Check sheet for the drawn part. Datum: minimum x, y, z corner. Units: mm. A direction names the side the tool comes from. Coordinates: 2 decimals unless noted, no trailing zeros. Write each loop counter-clockwise with the first axis right and the second up, starting at its lowest first coordinate (ties: lowest second). Pieces come first, ordered by that corner, then holes. Notation, with made-up numbers: (67.25, 63.5) - (96.25, 63.5) arc R17 ccw to (96.25, 84.5) - close; hole circle Ø6 at (63.25, 17.5). An arc over 180 degrees is marked (long way). Use CSV: the item, a comma, the result in double quotes. Start each with the question number.
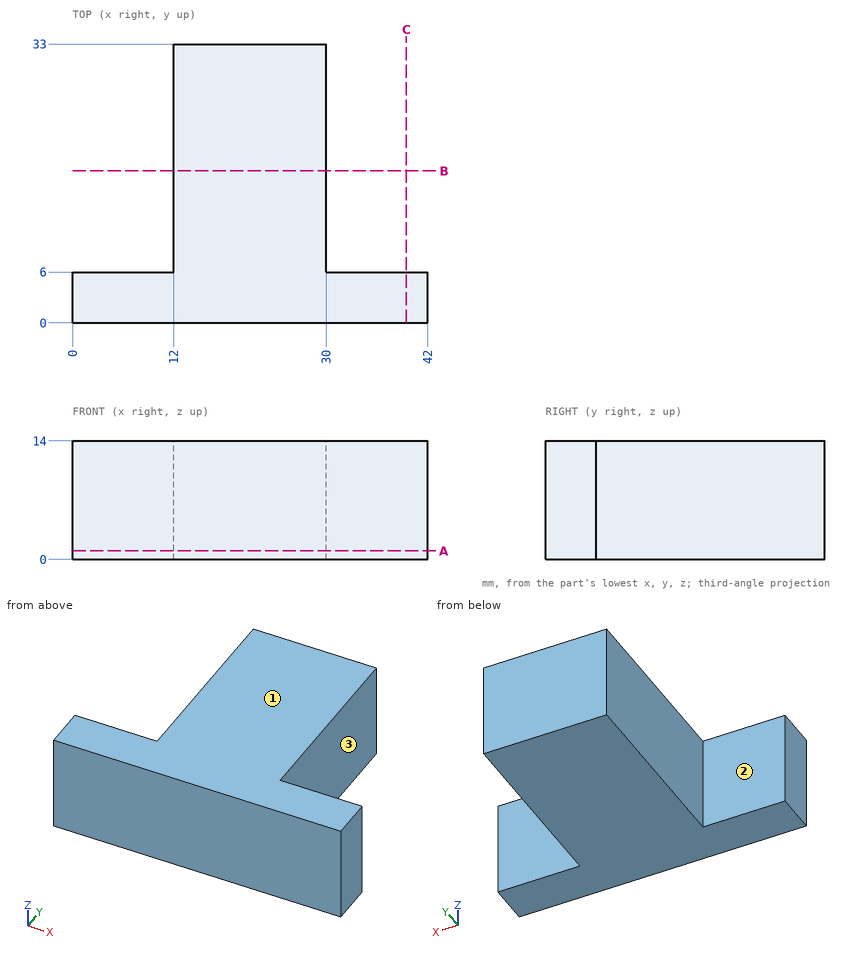
Q1. Scan lines: line 1 along Y through (x, z) = (3, 7); line 2 along X through (y, z) = (10.5, 3). Record each from-to range of solid material in increasing order. Write a range as from..to.
Q2. Gauge pin test, flat ends, axial feed: pin 1 (5 mm diameter, centred on x = 9, y = 24, fed in from +Z); pin 2 (2 mm diameter, centred on y = 19, z = 9, fed in from +X); pin 3 (3.5 mm diameter, centred on x = 9, z = 6.5, fed in from +Y). Record the tip position at first contact, or that the pin passes through.
Q3. Cross-section at C-C (x = 39.5). Record the cut outline in (y, z).
Q4. Tool access check on the marked faces 1, 2 and 3. Record the directions out of +Z, -Z, +X, -X, +Y, -Y that give a thin tool (end or side, any length) a straight path to the whole face; none if there is none.
Q5. Cross-section at B-B (y = 18). Record the cut outline in (x, z).
Q6. Cross-section at A-A (z = 1). Record the cut outline in (x, y).
Reply:
1,line 1,"0..6"
1,line 2,"12..30"
2,pin 1,"through"
2,pin 2,"x = 30"
2,pin 3,"y = 6"
3,outline,"(0, 0) - (6, 0) - (6, 14) - (0, 14) - close"
4,face 1,"+Z, +X, -X, +Y, -Y"
4,face 2,"+Z, -Z, -X, +Y"
4,face 3,"+Z, -Z, +X, +Y"
5,outline,"(12, 0) - (30, 0) - (30, 14) - (12, 14) - close"
6,outline,"(0, 0) - (42, 0) - (42, 6) - (30, 6) - (30, 33) - (12, 33) - (12, 6) - (0, 6) - close"
